For this review, use the dimensioned drawing (mm, ordinates from the lowest corner) and the shaded views. Round coordinates to 2 decimals unless told otherwise and drop trailing zeros. Loops run counter-clockwise (first coordinate to the right, second up) from the corner with the lowest first, then second, coordinate; pieces in that order, holes last. Notation, with made-up numbers: M -36.75,11 L -18.75,11 A18 ccw -18.75,36 Z; hole C 38,84.5 d10. An arc over 180 degrees is marked long. One line per item, written item: value. Start each with the question number.
Item 1: For line 1 along Y through (x, z) = (564.5, 11); line 2 along X through (y, z) = (186.5, 4.5), list the stretches that pass through material, from the lowest coordinate up.
Item 2: Clearance check with flat-ended pins moving along their axes: pin 1 (1.5 mm diameter, centred on y = 246, z = 2, fed in from +X); pin 2 (2 mm diameter, centred on x = 324.5, z = 9, fed in from +Y); pin 3 (6.5 mm diameter, centred on x = 6.5, z = 7.5, fed in from +Y). State where each tip first meets the part, or that it passes through.
Item 3: We need section A-A (y = 94). Write out the cut boundary in (x, z), then the cut area to 3 significant figures.
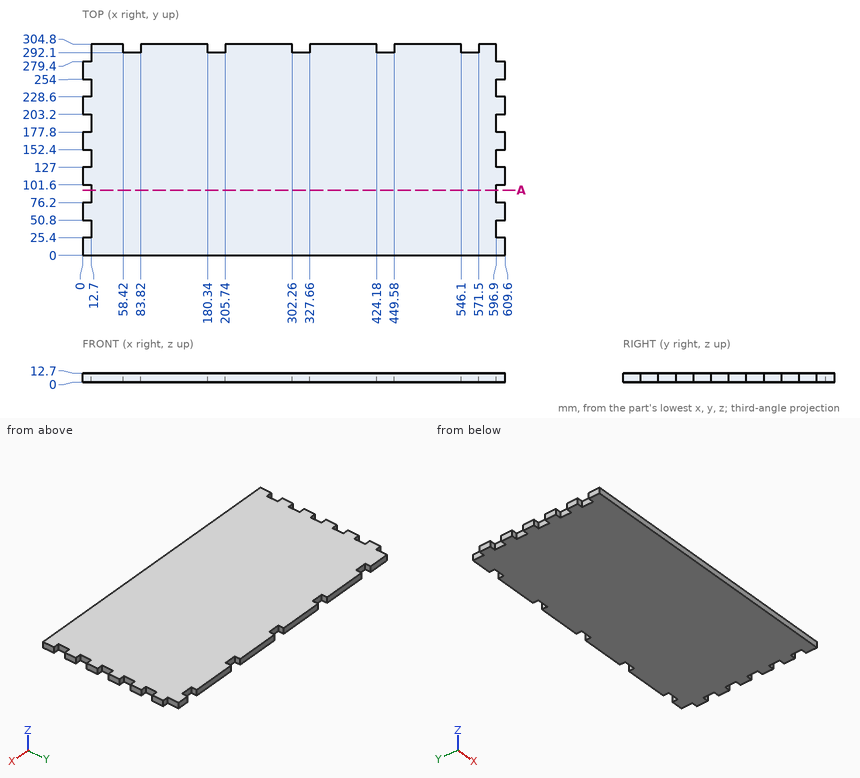
A:
1. line 1: 0 to 292.1
1. line 2: 12.7 to 596.9
2. pin 1: x = 596.9
2. pin 2: y = 292.1
2. pin 3: y = 279.4
3. outline: M 12.7,0 L 596.9,0 L 596.9,12.7 L 12.7,12.7 Z
3. area: 7,420 mm2
